The model under review builds one solid part; all positions refer to its coordinate system, in mm. Coordinates: 2 decimals unless noted, no trailing zeros. Order: outer loops, then holes, each group sorted by start corner. A loop starts at its lowest first (then second) coordinate and runs counter-clockwise, first axis right, second up. Notation, with made-up numbers: (74.25, 56.25) -> (87.25, 56.25) arc R28 ccw to (87.25, 88.25) -> close; hole circle Ø8 at (47.5, -25.75). An arc over 180 degrees is marked (long way). Use one line per item in the form item = value.
from build123d import *

# Parameters (mm, degrees)
F0_R     = 10.9855
F1_DEPTH = 25.4


with BuildPart() as f1:
    # F0 (on Front) → F1 (new body)
    with BuildSketch(Plane.XZ):
        with BuildLine():
            Line((44.12074, 16.901975), (20.145995, 17.604334))
            Line((20.145995, 17.604334), (23.131371, 15.880726))
            ThreePointArc((23.131371, 15.880726), (31.230244, 14.07893), (34.843798, 6.6103))
            ThreePointArc((34.843798, 6.6103), (32.05399, -0.124892), (25.318798, -2.9147))
            Line((25.318798, -2.9147), (25.318798, -14.617815))
            ThreePointArc((25.318798, -14.617815), (29.44571, -4.435593), (39.497305, 0))
            ThreePointArc((39.497305, 0), (39.657927, 9.039407), (44.12074, 16.901975))
        make_face()
        with BuildLine():
            Line((-23.131371, 15.880726), (-20.145995, 17.604334))
            Line((-20.145995, 17.604334), (-44.12074, 16.901975))
            ThreePointArc((-44.12074, 16.901975), (-39.657927, 9.039407), (-39.497305, 0))
            ThreePointArc((-39.497305, 0), (-29.44571, -4.435593), (-25.318798, -14.617815))
            Line((-25.318798, -14.617815), (-25.318798, -2.9147))
            ThreePointArc((-25.318798, -2.9147), (-34.77994, 7.711396), (-23.131371, 15.880726))
        make_face()
        with BuildLine():
            ThreePointArc((20.145995, 17.604334), (11.247841, 19.396708), (5.246522, 26.206549))
            add(Edge.make_bspline(
                [(-5.246522, 26.206549), (-4.375539, 14.018499), (0, 14.018499), (4.375539, 14.018499), (5.246522, 26.206549)],
                knots=[1.771192, 1.771192, 1.771192, 3.141593, 3.141593, 4.511993, 4.511993, 4.511993], degree=2, weights=[1, 0.774292, 1, 0.774292, 1]))
            ThreePointArc((-5.246522, 26.206549), (-11.247841, 19.396708), (-20.145995, 17.604334))
            Line((-20.145995, 17.604334), (-23.131371, 15.880726))
            ThreePointArc((-23.131371, 15.880726), (-17.850168, 12.521746), (-15.793798, 6.6103))
            ThreePointArc((-15.793798, 6.6103), (-18.583606, -0.124892), (-25.318798, -2.9147))
            Line((-25.318798, -2.9147), (-25.318798, -14.617815))
            ThreePointArc((-25.318798, -14.617815), (-19.310808, -13.551406), (-13.31532, -14.685998))
            ThreePointArc((-13.31532, -14.685998), (-4.759292, -20.223493), (0, -29.235629))
            ThreePointArc((0, -29.235629), (4.759292, -20.223493), (13.31532, -14.685998))
            ThreePointArc((13.31532, -14.685998), (19.310808, -13.551406), (25.318798, -14.617815))
            Line((25.318798, -14.617815), (25.318798, -2.9147))
            ThreePointArc((25.318798, -2.9147), (15.857655, 5.509205), (23.131371, 15.880726))
            Line((23.131371, 15.880726), (20.145995, 17.604334))
        make_face()
        Circle(F0_R, mode=Mode.SUBTRACT)
    extrude(amount=F1_DEPTH)


solid = f1.part
Item 1: We need section D-D (z = -23). Write out the cut boundary in (x, y), plus the area to 3 significant figures.
Results found:
outline = (-2.63, -25.4) -> (2.63, -25.4) -> (2.63, 0) -> (-2.63, 0) -> close
area = 134 mm²
Item 2: Clearance check with flat-ended pins moving along their axes: pin 1 (1 mm diameter, centred on x = -32, y = -22.5, fed in from -Z); pin 2 (8 mm diameter, centred on x = -11.5, y = -4.5, fed in from -Z); pin 3 (1 mm diameter, centred on x = -4, y = -11.5, fed in from -Z). State where each tip first meets the part, or that it passes through.
Results found:
pin_1 = -2.68
pin_2 = -17.73
pin_3 = -21.74
Item 3: To check wall thickness, follow L1, parallel to X at y = -24, z = -1.5; L2, parallel to X at y = -6, z = 23; L3, parallel to Z at x = -17.5, y = -10.5. State the ranges of each line that lie inside material, in increasing order. Write a range as from..to.
Results found:
L1 = -33.48..-30.31, -20.32..-10.88, 10.88..20.32, 30.31..33.48
L2 = -7.12..-4.88, 4.88..7.12
L3 = -13.66..1.17, 12.05..17.52
Item 4: We need section C-C (y = -2.5). State how many separate pieces and enclosed holes the cut face has, plus the area to 3 significant figures.
Results found:
separate_pieces = 1
enclosed_holes = 3
area = 1,450 mm²
Item 5: Draft analysis for pull direction X (two halves, no side actions). For faces 1 (the face through (-19.4, -12.52, -13.55)), 2 (the face through (4.66, -12.52, -20.33)), 3 (the face through (-39.69, -12.52, 9.16)), 4 (the face through (11.36, -12.522, 19.333)), state which applies: released by +X, released by -X, zero draft, split by the parting line, or undercut.
Results found:
face_1 = undercut
face_2 = released by +X
face_3 = released by -X
face_4 = undercut
Item 6: We need section B-B (x = -8). Write out the cut boundary in (y, z).
Results found:
outline = (-25.4, -17.37) -> (0, -17.37) -> (0, -7.53) -> (-25.4, -7.53) -> close; (-25.4, 7.53) -> (0, 7.53) -> (0, 21.97) -> (-25.4, 21.97) -> close
Item 7: We need section A-A (z = -8.5). Write out the cut boundary in (x, y), plus the area to 3 significant figures.
Results found:
outline = (-26.66, -25.4) -> (-6.96, -25.4) -> (-6.96, 0) -> (-26.66, 0) -> close; (6.96, -25.4) -> (26.66, -25.4) -> (26.66, 0) -> (6.96, 0) -> close
area = 1,000 mm²
